For this review, use the dimensioned drawing (mm, ordinates from the lowest corner) and the shaded views. A direction names the side the tool comes from. Give positions to 0.01 mm unless a question says otherwise; leave off trailing zeros. Order: outer loops, then holes, each group sorted by start corner. A loop starts at its lowest first (then second) coordinate and runs counter-clockwise, first axis right, second up. Notation, with made-up numbers: (33, 21.5) - (64, 21.5) arc R9 ccw to (64, 33.5) - close; hole circle Ø6 at (-18.75, 48.25). An arc over 180 degrees is marked (long way). One line per item, written item: value.
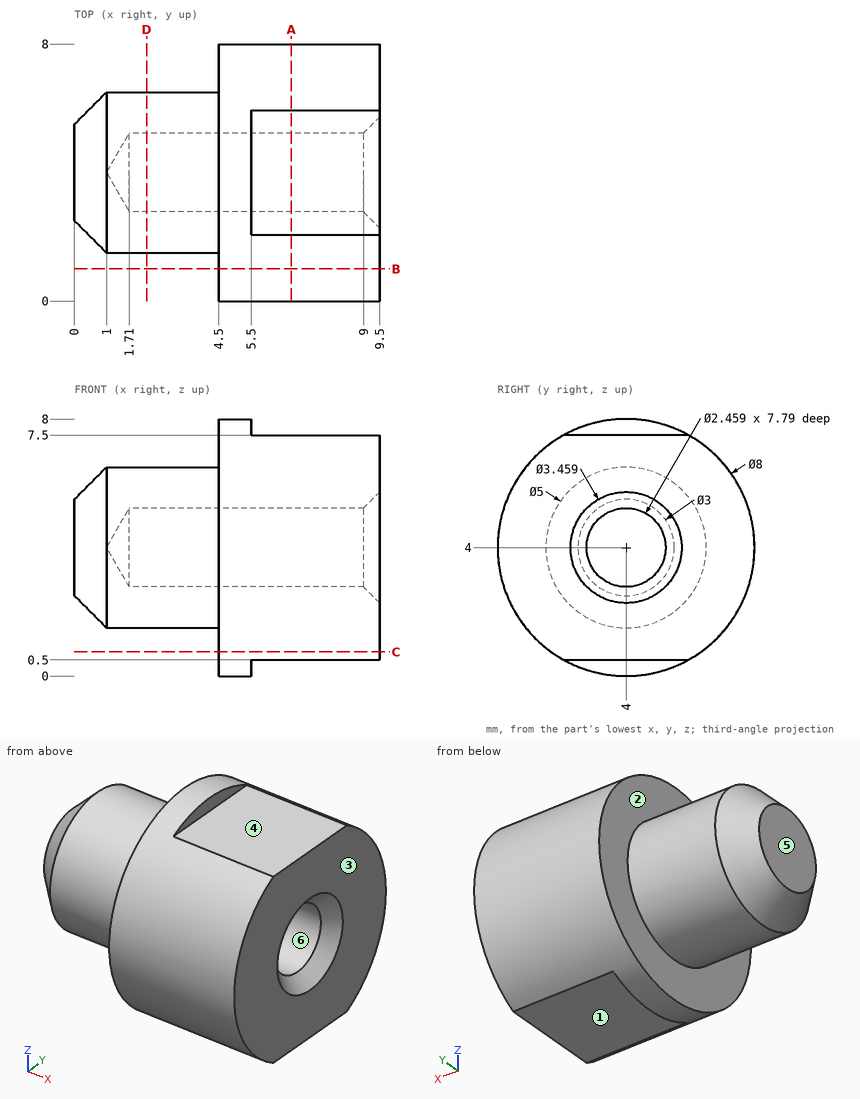
(1) Draft analysis for pull direction Z (two halves, no side actions). For the marked faces 4, 5 and 6, state which applies: pulls with the +Z half, pulls with the -Z half, needs draft (parallel to the pull), parting line crosses it, or undercut.
Answers below:
face 4: pulls with the +Z half
face 5: needs draft
face 6: undercut
(2) Take a section at D-D (x = 2.25). Write out the cut boundary in (y, z).
Answers below:
outline: circle Ø5 at (4, 4); hole circle Ø2.46 at (4, 4)
(3) Take a section at C-C (z = 0.75). Write out the cut boundary in (x, y).
Answers below:
outline: (4.5, 1.67) - (9.5, 1.67) - (9.5, 6.33) - (4.5, 6.33) - close
(4) Take a section at A-A (x = 6.75). Write out the cut boundary in (y, z).
Answers below:
outline: (2.06, 0.5) - (5.94, 0.5) arc R4 ccw to (5.94, 7.5) - (2.06, 7.5) arc R4 ccw to start; hole circle Ø2.46 at (4, 4)
(5) For P1, Ø1.2, axis at x = 7, y = 3, coming from the -Z side; P2, Ø1.5, axis at x = 8, z = 1.5, coming from the -Y side, all flat-tipped, find the tip position at first contact; note any pin that passes through.
Answers below:
P1: stops at z = 0.5
P2: stops at y = 0.4
(6) Take a section at B-B (y = 1). Write out the cut boundary in (x, z).
Answers below:
outline: (4.5, 1.35) - (9.5, 1.35) - (9.5, 6.65) - (4.5, 6.65) - close
(7) Wall thickness on line 1 (Y direction, x = 6.75, z = 4); line 2 (Z direction, x = 7, y = 4); line 3 (X direction, y = 5.5, z = 6.75): over which ranges is each line inside the solid? List them lowest first. Write a range as from..to.
Answers below:
line 1: y = 0..2.77, 5.23..8
line 2: z = 0.5..2.77, 5.23..7.5
line 3: x = 4.5..9.5
(8) Machinability: for the marked faces 1, 2 and 3, which of the approach directions +Z, -Z, +X, -X, +Y, -Y give a long, thin tool a straight path to every point of the face, cutting with its end or side? Answer none if there is none.
Answers below:
face 1: -Z, +X, +Y, -Y
face 2: -X
face 3: +Z, -Z, +X, +Y, -Y
